Print and shaded views of the part. All mm, measured from the part's lowest x, y and z. A direction names the side the tool comes from. Round coordinates to 2 decimals unless told otherwise and drop trailing zeros. Loops run counter-clockwise (first coordinate to the right, second up) from the corner with the lowest first, then second, coordinate; pieces in that order, holes last. Notation, with made-up numbers: (25.5, 82) - (67.5, 82) arc R8 ccw to (67.5, 96) - close; hole circle Ø5 at (22.5, 16). An arc over 180 degrees is marked (long way). Use one line per item in the form item = value.
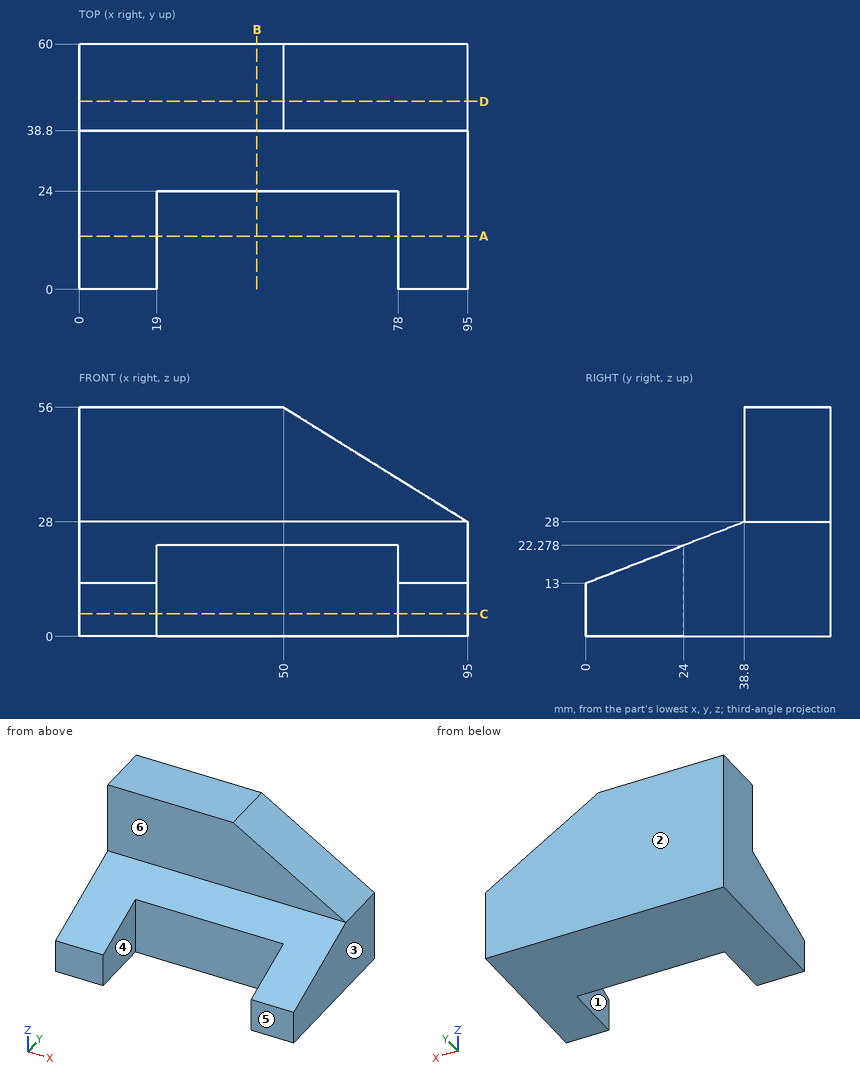
1. Pull direction X, two halves, no side cores. Call the marked faces 1, 2 and 3: +X half, -X half, draft (parallel to the pull), parting line (faces both ways), or undercut.
Geometry check:
face_1 = undercut
face_2 = draft
face_3 = +X half
2. Cut at C-C, the plane z = 5.5. Give the cut face in (x, y).
Geometry check:
outline = (0, 0) - (19, 0) - (19, 24) - (78, 24) - (78, 0) - (95, 0) - (95, 60) - (0, 60) - close
3. Wall check: probe 1 along X at (y, z) = (5, 5); probe 2 along Y at (x, z) = (20.5, 51); probe 3 along Y at (x, z) = (44, 12.5). Give the ranges that are in metal, low to high.
Geometry check:
probe_1 = 0 to 19, 78 to 95
probe_2 = 38.8 to 60
probe_3 = 24 to 60
4. Cut at D-D, the plane y = 46. Give the cut face in (x, z).
Geometry check:
outline = (0, 0) - (95, 0) - (95, 28) - (50, 56) - (0, 56) - close
5. Tool access for the marked faces 4, 5 and 6: list every direction of +Z, -Z, +X, -X, +Y, -Y with a clear straight run to the whole face (end or side of a thin tool).
Geometry check:
face_4 = +Z, -Z, -Y
face_5 = +Z, -Z, +X, -X, -Y
face_6 = +Z, +X, -X, -Y
6. Cut at B-B, the plane x = 43.5. Give the cut face in (y, z), plus the area to 3 significant figures.
Geometry check:
outline = (24, 0) - (60, 0) - (60, 56) - (38.8, 56) - (38.8, 28) - (24, 22.28) - close
area = 1,560 mm^2
7. Flat gauge pins, fed straight in: pin 1 (2 mm diameter, centred on x = 19.5, z = 38.5, fed in from -Y); pin 2 (11 mm diameter, centred on x = 59.5, z = 9.5, fed in from -Y). Where does each tip first touch, or does it go through?
Geometry check:
pin_1 = 38.8
pin_2 = 24
8. Cut at A-A, the plane y = 13. Give the cut face in (x, z) (1 decimal), plus the area to 3 significant figures.
Geometry check:
outline = (0, 0) - (19, 0) - (19, 18) - (0, 18) - close; (78, 0) - (95, 0) - (95, 18) - (78, 18) - close
area = 649 mm^2
